Build history of the part. All positions in model axes, mm. Face numbers are marked on the shaded views. Give positions to 0.01 mm unless a question says otherwise; leave off trailing zeros. Order: outer loops, then holes, each group sorted by start corner. A loop starts at its lowest first (then second) coordinate and runs counter-clockwise, first axis right, second up. Notation, with made-up numbers: M 41.25,65 L 68.25,65 A27 ccw 68.25,81 Z; hole C -17.5,43.25 d8. An arc over 180 degrees is marked long. One line per item, written item: value.
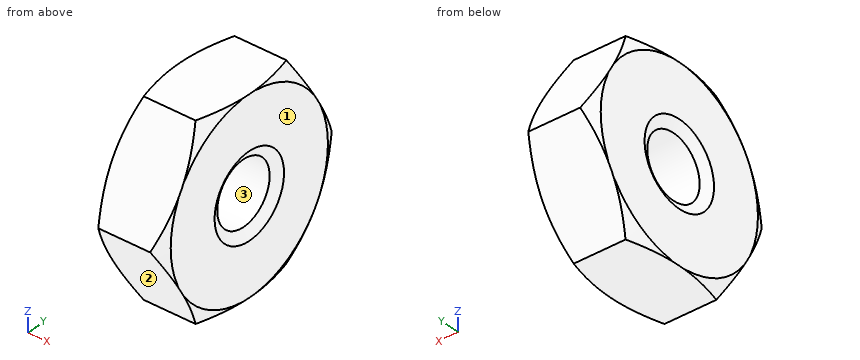
Autodesk Inventor part; units mm, degrees
ref_plane "Work Plane1" through (-9.5512, 0, 0) normal (0, -0.866, -0.5) x (1, 0, 0)
ref_plane "YZ Plane" through (0, 0, 0) normal (1, 0, 0) x (0, 1, 0)
ref_plane "XZ Plane" through (0, 0, 0) normal (0, 1, 0) x (-1, 0, 0)
sketch "Sketch1" plane through (0, 0, 0) normal (1, 0, 0) x (0, 1, 0)
  line L0 (-4.5754, 0) -> (-2.2877, 3.9624)
  line L1 (-2.2877, 3.9624) -> (2.2877, 3.9624)
  line L2 (2.2877, 3.9624) -> (4.5754, 0)
  line L3 (4.5754, 0) -> (2.2877, -3.9624)
  line L4 (2.2877, -3.9624) -> (-2.2877, -3.9624)
  line L5 (-2.2877, -3.9624) -> (-4.5754, 0)
  point P0 (0, 0)
  point P1 (0, 0)
  dimension "d0" = 9.1508
extrude "Body" add sketch "Sketch1" along normal blind 2.8956
sketch "Sketch2" plane through (0, 0, 0) normal (0, 0, 1) x (1, 0, 0)
  line L0 (0, 2.2877) -> (0, 4.5754)
  line L1 (0, 4.5754) -> (2.8956, 4.5754)
  line L2 (2.8956, 2.2877) -> (2.8956, 4.5754)
  line L3 (-0.5791, 0) -> (3.4747, 0)
  line L4 (0.3539, 4.5754) -> (0, 3.9624)
  line L5 (2.5417, 4.5754) -> (2.8956, 3.9624)
  dimension "d3" = 30
  dimension "d4" = 30
  dimension "d5" = 7.9248
  dimension "d6" = 7.9248
revolve "Chamfer1" cut sketch "Sketch2" angle 360 about axis through (-10, 0, 0) along (1, 0, 0)
sketch "Sketch3" plane through (2.8956, 0, 0) normal (1, 0, 0) x (0, 0, -1)
  arc A0 (-1.9812, -3.4315) -> (1.9812, -3.4315) centre (0, 0) ccw
hole "Thread" at (2.8956, 0, 0) direction (-1, 0, 0) diameter 2.6416 end through all
chamfer "Chamfer2" distance 0.4296 angle 30 1 edges at (2.8956, 0, 1.3208) measured on face at (2.8956, 3.0642, -0.0531)
chamfer "Chamfer3" distance 0.4296 angle 30 1 edges at (0, 0, 1.3208) measured on face at (0, -3.0642, -0.0531)
ref_plane "Work Plane1" through (-9.5512, 0, 0) normal (0, -0.866, -0.5) x (1, 0, 0)
equation "\"d0\" = 1.1547 * SW"
equation "\"d1\" = KOH"
equation "\"d3\" = ANG1"
equation "\"d4\" = ANG2"
equation "\"d5\" = SW0"
equation "\"d6\" = SW01"
equation "\"d8\" = -0.5 * GD1 + 0.5 * NND"
equation "\"d40\" = -0.5 * GD1 + 0.5 * NND"
equation "\"d10\" = -0.5 * GD1 + 0.5 * NND"
equation "\"d41\" = -0.5 * GD1 + 0.5 * NND"
equation "\"ANG1\" = 30deg"
equation "\"ANG2\" = 30deg"
equation "\"NND\" = 3.5052"
equation "\"KOH\" = 2.8956"
equation "\"SW\" = 7.9248"
equation "\"SW0\" = SW"
equation "\"SW01\" = SW"
equation "\"THREADDIA\" = 3.5052"
equation "\"TOA\" = 30deg"
equation "\"E0\" = 1.155 * SW"
properties part number "ANSI B18.2.2 - 6 - 32" material "Steel, Mild"
1) Pin check, flat tip, straight feed: pin 1 (1.6 mm diameter, centred on y = 0, z = 0, fed in from -X). Stop position of the tip, or through.
Check values:
pin 1: through
2) Drill centre lines: probe 1 along Z at (x, y) = (0.9, 0); probe 2 along Z at (x, y) = (2.2, 0.5); probe 3 along Y at (x, z) = (1.95, -1). Where is each one in solid material? Low to high. Write a range as from..to.
Check values:
probe 1: -3.96..-1.32, 1.32..3.96
probe 2: -3.96..-1.22, 1.22..3.96
probe 3: -4..-0.86, 0.86..4
3) Saw through at A-A, the plane x = 0.85. Write the cut outline in (y, z).
Check values:
outline: M -4.58,0 L -2.29,-3.96 L 2.29,-3.96 L 4.58,0 L 2.29,3.96 L -2.29,3.96 Z; hole C 0,0 d2.64
4) Mould opens along Y. For the marked faces 1, 2 and 3 say: released by +Y, released by -Y, zero draft, split by the parting line, or undercut.
Check values:
face 1: zero draft
face 2: released by -Y
face 3: undercut
